Design review of the part built by this model. Coordinates are the model's own, in mm. A direction names the side the tool comes from. Coordinates: 2 decimals unless noted, no trailing zeros. Order: outer loops, then holes, each group sorted by start corner. A loop starts at its lowest first (then second) coordinate and runs counter-clockwise, first axis right, second up. Notation, with made-up numbers: (13, -35.75) -> (47, -35.75) arc R24 ccw to (47, -1.75) -> close; hole circle Ø6 at (62.25, 1). An arc over 180 degrees is marked (long way). Use a Markdown table: item, result. Add a question column.
Q1. Machinability: for faces 1 (the face through (13.5, 4.49, 0.07)), 2 (the face through (25, 0, 4)), which of the approach directions +Z, -Z, +X, -X, +Y, -Y give a long, thin tool a straight path to every point of the face, cutting with its end or side? Answer none if there is none.
Q2. Add section B-B (x = 5). State the section outline as (y, z) points.
Q3. Add section D-D (x = 26). State the section outline as (y, z) points, then the cut area to 3 significant figures.
Q4. Add section A-A (y = 0). State the section outline as (x, z) points.
Q5. Insertion check: pin 1 (3.5 mm diameter, centred on x = 35, z = 0, fed in from -Y). The pin has a flat end and moves straight along its axis. Give the tip position at first contact, or say it passes through.
Q6. The part is to be moulded in two halves that separate along Z. For faces 3 (the face through (43.5, 0.07, 4.51)), 4 (the face through (25, 0, -5)), 5 (the face through (33.8, -4.5, -0.9)), say which applies: pulls with the +Z half, pulls with the -Z half, needs draft (parallel to the pull), parting line crosses it, or undercut.
Q7. Wall thickness on probe 1 along Y at (x, z) = (10, -1.25); probe 2 along Y at (x, z) = (45, 4.3): over which ranges is each line inside the solid? List them lowest first.
Q8. Add section C-C (z = 3). State the section outline as (x, y) points.
Autodesk Inventor part; units mm, degrees
ref_plane "YZ Plane" through (0, 0, 0) normal (1, 0, 0) x (0, 1, 0)
ref_plane "XZ Plane" through (0, 0, 0) normal (0, 1, 0) x (-1, 0, 0)
ref_plane "XY Plane" through (0, 0, 0) normal (0, 0, 1) x (1, 0, 0)
sketch "スケッチ1" plane through (0, 0, 0) normal (1, 0, 0) x (0, 1, 0)
  line L0 (5, 5) -> (-5, 5)
  line L1 (-5, 5) -> (-5, -5)
  line L2 (-5, -5) -> (5, -5)
  line L3 (5, -5) -> (5, 5)
  line L4 (4, 4) -> (-4, 4)
  line L5 (-4, 4) -> (-4, -4)
  line L6 (-4, -4) -> (4, -4)
  line L7 (4, -4) -> (4, 4)
  point P0 (0, 0)
  dimension "d0" = 1
  dimension "d1" = 1
  dimension "d2" = 1
  dimension "d3" = 1
  dimension "d4" = 10
  dimension "d5" = 10
  dimension "d6" = 5
  dimension "d7" = 5
extrude "押し出し1" add sketch "スケッチ1" along normal blind 50
sketch "スケッチ2" plane through (0, -5, 5) normal (0, 0, 1) x (1, 0, 0)
  circle A0 centre (5, 5) radius 1.5
  line L0 (0, 10) -> (0, 0)
  line L1 (0, 0) -> (50, 0)
  circle A1 centre (45, 5) radius 1.5
  line L2 (50, 10) -> (50, 0)
  point P0 (0, 5)
  dimension "d10" = 3
  dimension "d11" = 5
  dimension "d12" = 5
  dimension "d13" = 5
  dimension "d14" = 5
  dimension "d15" = 3
sketch "スケッチ3" plane through (0, -5, -5) normal (0, -1, 0) x (1, 0, 0)
  circle A0 centre (15, 5) radius 1.5
  line L0 (0, 10) -> (0, 0)
  line L1 (0, 10) -> (50, 10)
  circle A1 centre (35, 5) radius 1.5
  line L2 (50, 10) -> (50, 0)
  line L3 (0, 0) -> (50, 0)
  point P0 (0, 5)
  dimension "d16" = 3
  dimension "d17" = 15
  dimension "d18" = 5
  dimension "d19" = 15
  dimension "d20" = 5
  dimension "d21" = 3
extrude "押し出し2" cut sketch "スケッチ2" against normal blind 50
extrude "押し出し3" cut sketch "スケッチ3" against normal blind 50 contours A0 | A1
properties part number "角パーツ" material "アルミニウム 6061"
Established:
| question | item | result |
|---|---|---|
| 1 | face 1 | +Y, -Y |
| 1 | face 2 | +X, -X |
| 2 | outline | (-5, -5) -> (-1.5, -5) -> (-1.5, -4) -> (-4, -4) -> (-4, 4) -> (-1.5, 4) -> (-1.5, 5) -> (-5, 5) -> close; (1.5, -5) -> (5, -5) -> (5, 5) -> (1.5, 5) -> (1.5, 4) -> (4, 4) -> (4, -4) -> (1.5, -4) -> close |
| 3 | outline | (-5, -5) -> (5, -5) -> (5, 5) -> (-5, 5) -> close; hole (-4, -4) -> (4, -4) -> (4, 4) -> (-4, 4) -> close |
| 3 | area | 36.0 mm^2 |
| 4 | outline | (0, -5) -> (3.5, -5) -> (3.5, -4) -> (0, -4) -> close; (0, 4) -> (3.5, 4) -> (3.5, 5) -> (0, 5) -> close; (6.5, -5) -> (43.5, -5) -> (43.5, -4) -> (6.5, -4) -> close; (6.5, 4) -> (43.5, 4) -> (43.5, 5) -> (6.5, 5) -> close; (46.5, -5) -> (50, -5) -> (50, -4) -> (46.5, -4) -> close; (46.5, 4) -> (50, 4) -> (50, 5) -> (46.5, 5) -> close |
| 5 | pin 1 | y = -5 |
| 6 | face 3 | needs draft |
| 6 | face 4 | pulls with the -Z half |
| 6 | face 5 | undercut |
| 7 | probe 1 | -5 to -4, 4 to 5 |
| 7 | probe 2 | -5 to -1.5, 1.5 to 5 |
| 8 | outline | (0, -5) -> (50, -5) -> (50, -4) -> (0, -4) -> close; (0, 4) -> (50, 4) -> (50, 5) -> (0, 5) -> close |
